from build123d import *

# Parameters (mm, degrees)
F1_DEPTH = 80
F3_DEPTH = 25
F4_R     = 39.99999
F6_R     = 10
F7_DEPTH = 101.1
F8_R     = 10


# Not quite as in the source:
# - a fillet or chamfer is up to 0.001 mm smaller than in the source, because OpenCascade refuses the exact size


with BuildPart() as f1:
    # F0 (on Top) → F1 (new body)
    with BuildSketch(Plane.XY):
        Polygon((-75.6232507176, 0), (74.3767492824, 0), (74.3767492824, 10), (-35.9964989842, 10), (-74.7411806087, 89.4383695755), (-83.7291210717, 85.0546581076), (-57.4268522644, 31.1270153297), (-75.4027331904, 22.3595923939), (-101.7050019977, 76.2872351718), (-110.6929424607, 71.9035237039), align=None)
    extrude(amount=F1_DEPTH)

    # F2 (on face) → F3 (cut)
    with BuildSketch(Plane(origin=(0, 10, 0), x_dir=(-1, 0, 0), z_dir=(0, 1, 0))):
        with BuildLine():
            ThreePointArc((-14.3767492824, 50), (-24.3767492824, 40), (-14.3767492824, 30))
            Line((-14.3767492824, 30), (-14.3767492824, 50))
        make_face()
        with BuildLine():
            Line((-134.3767492824, 30), (-14.3767492824, 30))
            ThreePointArc((-14.3767492824, 30), (-24.3767492824, 40), (-14.3767492824, 50))
            Line((-14.3767492824, 50), (-134.3767492824, 50))
            Line((-134.3767492824, 50), (-134.3767492824, 30))
        make_face()
        with BuildLine():
            Line((-14.3767492824, 50), (-14.3767492824, 30))
            ThreePointArc((-14.3767492824, 30), (-7.3056814706, 32.9289321881), (-4.3767492824, 40))
            ThreePointArc((-4.3767492824, 40), (-7.3056814706, 47.0710678119), (-14.3767492824, 50))
        make_face()
    extrude(amount=-F3_DEPTH, mode=Mode.SUBTRACT)

    # F4 (radius 40 in the source; OpenCascade refuses exactly that, so slightly less here)
    f4_edges = [f1.edges().sort_by_distance(p)[0] for p in [
        (-79.235151, 87.246514, 80),
        (-106.198972, 74.095379, 80),
        (-106.198972, 74.095379, 0),
        (-79.235151, 87.246514, 0),
    ]]
    fillet(f4_edges, radius=F4_R)

    # F6 (on face) → F7 (cut)
    with BuildSketch(Plane(origin=(-25.1390245597, -12.2611215225, 0), x_dir=(-0.4383711468, 0.8987940463, 0), z_dir=(0.8987940463, 0.4383711468, 0))):
        with Locations((77.0729333162, 42.9970733821)):
            Circle(F6_R)
    extrude(amount=-F7_DEPTH, mode=Mode.SUBTRACT)

    # F8
    f8_edges = [f1.edges().sort_by_distance(p)[0] for p in [
        (74.376749, 5, 80),
        (74.376749, 5, 0),
    ]]
    fillet(f8_edges, radius=F8_R)


solid = f1.part
CAD build for the part. Positions are in the model's coordinates, mm. A direction names the side the tool comes from. Coordinates: 2 decimals unless noted, no trailing zeros. Write each loop counter-clockwise with the first axis right and the second up, starting at its lowest first coordinate (ties: lowest second). Pieces come first, ordered by that corner, then holes. Notation, with made-up numbers: M 79.5,35 L 96.5,35 A10 cw 96.5,44 Z; hole C 75.25,77 d6. An arc over 180 degrees is marked long. Return JSON: item names as keys, results as strings.
Item 1: Slice it at D-D, the plane z = 27.5. Write the cut outline in (x, y).
Findings below:
{"outline": "M -109.81,70.1 L -75.62,0 L 74.38,0 L 74.38,10 L -36,10 L -73.86,87.64 L -82.85,83.25 L -57.43,31.13 L -75.4,22.36 L -100.83,74.49 Z"}
Item 2: Slice it at C-C, the plane x = -1. Write the cut outline in (y, z).
Findings below:
{"outline": "M 0,0 L 10,0 L 10,80 L 0,80 Z"}
Item 3: Probe line 1 (Y direction, x = -55.5, z = 13); line 2 (Y direction, x = -73.5, z = 7); line 3 (Y direction, x = -21, z = 4.5). List the from-to ranges inside material, lowest first. Write a range as from..to.
Findings below:
{"line 1": "y = 0..49.99", "line 2": "y = 0..23.29, 64.08..70.69", "line 3": "y = 0..10"}
Item 4: Drop flat-ended pins along their axis: pin 1 Ø10 at (y, z) = (80.5, 55) entering from +X; pin 2 Ø4 at (x, z) = (-84.5, 15) entering from +Y; pin 3 Ø8 at (y, z) = (56, 31.5) entering from +X. Give the stop position or say it passes through.
Findings below:
{"pin 1": "stops at x = -67.94", "pin 2": "stops at y = 45.11", "pin 3": "stops at x = -56.48"}
Item 5: Slice it at B-B, the plane z = 48. Write the cut outline in (x, y), and give its area (3 significant figures).
Findings below:
{"outline": "M -110.34,71.18 L -98.67,47.26 L -89.69,51.64 L -101.35,75.56 Z; M -91.08,31.69 L -75.62,0 L 8.38,0 L 8.38,10 L -36,10 L -55.13,49.23 L -64.12,44.85 L -57.43,31.13 L -75.4,22.36 L -82.09,36.08 Z; M -83.37,84.33 L -71.71,60.41 L -62.72,64.79 L -74.39,88.71 Z", "area": "2,450 mm2"}
Item 6: Which spindle directions (+Z, -Z, +X, -X, +Y, -Y) get a long thin tool onto all of the face, cutting with end or side? Do faces 5 (the flat face through (-67.84, 52.48, 30.55)), 6 (the flat face through (44, 5, 50)), 7 (the flat face through (8, 10, 31)). Say none if no direction does.
Findings below:
{"face 5": "+Z, -Z", "face 6": "+X, +Y, -Y", "face 7": "+Z, -Z, +X, +Y"}
Item 7: Two-plate mould, pull along Y, no slides. Class faces 1 (the flat face through (-66.3, 26.8, 39.4)), 2 (the cylindrical face through (-58.98, 45.87, 43.44)), 3 (the flat face through (45, 5, 30)), 4 (the flat face through (-50.793, 40.337, 39.44)): +Y half, -Y half, draft (parallel to the pull), parting line (faces both ways), or undercut.
Findings below:
{"face 1": "undercut", "face 2": "undercut", "face 3": "draft", "face 4": "+Y half"}
Item 8: Slice it at A-A, the plane x = 37.5. Write the cut outline in (y, z).
Findings below:
{"outline": "M 0,0 L 10,0 L 10,30 L 0,30 Z; M 0,50 L 10,50 L 10,80 L 0,80 Z"}
